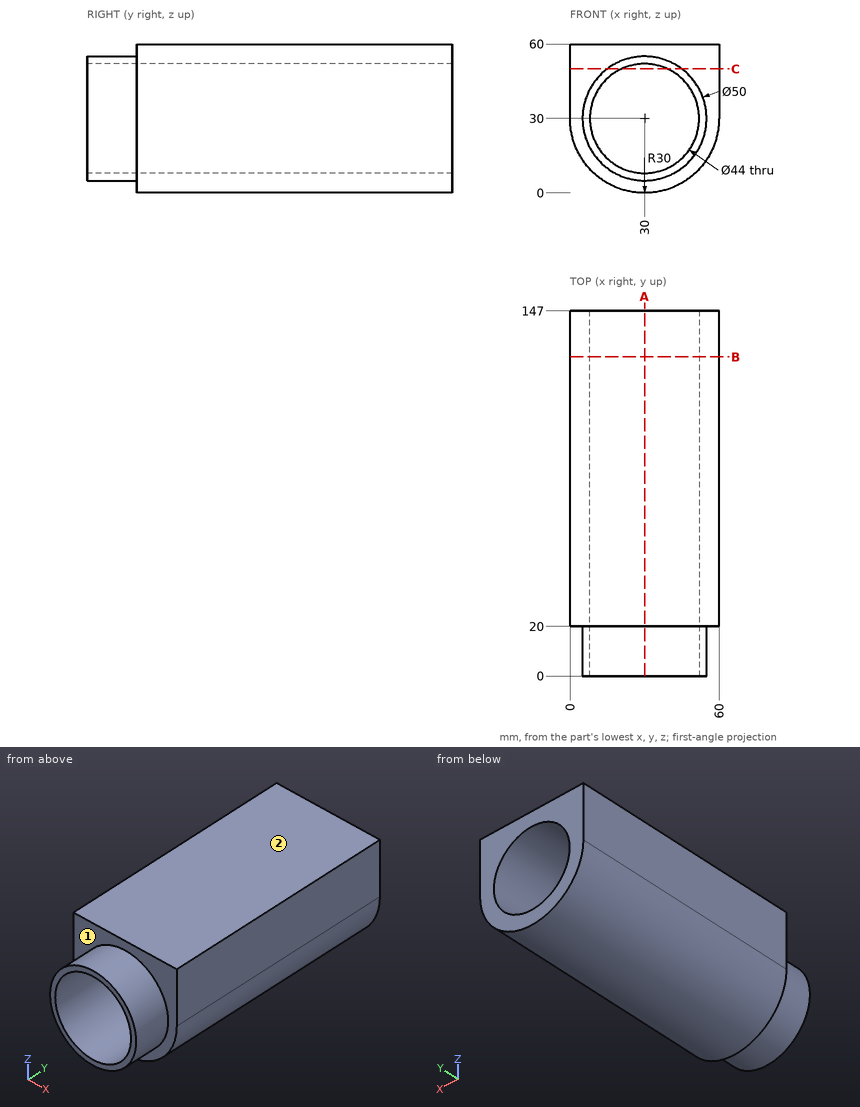
Here's the drawing with two shaded views (mm, measured from the low corner). I have some questions. A direction names the side the tool comes from. Give positions to 0.01 mm unless a question says otherwise; leave off trailing zeros. Write each loop counter-clockwise with the first axis right and the second up, starting at its lowest first coordinate (ties: lowest second). Pieces come first, ordered by that corner, then holes. Notation, with made-up numbers: (0, 51) - (34, 51) arc R29 cw to (34, 81) - close; hole circle Ø10 at (-22.5, 20.5). An arc over 180 degrees is marked (long way). Write item = value, one per line. Start each with the question number.
1. Imagine slicing it at A-A (x = 30). Please give me the cut outline in (y, z), and give its area (3 significant figures).
2. Imagine slicing it at B-B (y = 128.5). Please give me the cut outline in (x, z).
3. On a 3-axis mill with a long thin cutter (end or side, diameter ignored), from which of +Z, -Z, +X, -X, +Y, -Y can I reach the whole of each face in a straight line? I mean the marked faces 1 and 2. Say none if no direction works.
4. Imagine slicing it at C-C (z = 50). Please give me the cut outline in (x, y), and give its area (3 significant figures).
5. Please list where these lines run through material, in increasing order: line 1 (X direction, y = 50, z = 30); line 2 (Y direction, x = 35.5, z = 3.5).
6. For pin 1 (5 mm diameter, centred on x = 18, y = 48, fed in from -Z); pin 2 (10 mm diameter, centred on x = 28.5, y = 99, fed in from -Z), each with a flat end and sliding along its axis, tell me the tip position at first contact or that it passes through.
Worked answers:
q1.outline = (0, 5) - (20, 5) - (20, 0) - (147, 0) - (147, 8) - (0, 8) - close; (0, 52) - (147, 52) - (147, 60) - (20, 60) - (20, 55) - (0, 55) - close
q1.area = 2,150 mm2
q2.outline = (0, 30) arc R30 ccw to (60, 30) - (60, 60) - (0, 60) - close; hole circle Ø44 at (30, 30)
q3.face_1 = -Y
q3.face_2 = +Z, +X, -X, +Y, -Y
q4.outline = (0, 20) - (15, 20) - (15, 0) - (20.83, 0) - (20.83, 147) - (0, 147) - close; (39.17, 0) - (45, 0) - (45, 20) - (60, 20) - (60, 147) - (39.17, 147) - close
q4.area = 5,530 mm2
q5.line_1 = 0 to 8, 52 to 60
q5.line_2 = 20 to 147
q6.pin_1 = 1.54
q6.pin_2 = 0
